Autodesk Inventor part; units mm, degrees
ref_plane "YZ Plane" through (0, 0, 0) normal (1, 0, 0) x (0, 1, 0)
ref_plane "XZ Plane" through (0, 0, 0) normal (0, 1, 0) x (-1, 0, 0)
ref_plane "XY Plane" through (0, 0, 0) normal (0, 0, 1) x (1, 0, 0)
sketch "Skizze1" plane through (0, 0, 0) normal (0, 1, 0) x (-1, 0, 0)
  line L0 (47, -24.5) -> (-47, -24.5)
  line L1 (-47, -24.5) -> (-47, 24.5)
  line L2 (-47, 24.5) -> (47, 24.5)
  line L3 (47, 24.5) -> (47, -24.5)
  point P0 (0, 0)
  point P1 (0, -24.5)
  point P2 (47, 0)
  dimension "d0" = 49
  dimension "d1" = 94
extrude "Extrusion1" add sketch "Skizze1" along normal blind 2
sketch "Skizze2" plane through (0, 2, 0) normal (0, 1, 0) x (1, 0, 0)
  circle A0 centre (-43.5, 21) radius 1.75
  circle A1 centre (-43.5, -21) radius 1.75
  circle A2 centre (43.5, -21) radius 1.75
  circle A3 centre (43.5, 21) radius 1.75
  point P0 (0, 0)
  dimension "d4" = 3.5
  dimension "d5" = 3.5
  dimension "d6" = 3.5
  dimension "d7" = 3.5
  dimension "d8" = 87
  dimension "d9" = 43.5
  dimension "d10" = 42
  dimension "d11" = 21
extrude "Extrusion2" cut sketch "Skizze2" against normal through all
sketch "Skizze4" plane through (0, 2, 0) normal (0, 1, 0) x (1, 0, 0)
  line L0 (-39.5, 24) -> (39.5, 24)
  line L1 (46.5, 17) -> (46.5, -17)
  line L2 (39.5, -24) -> (-39.5, -24)
  line L3 (-46.5, -17) -> (-46.5, 17)
  line L4 (47, -24.5) -> (47, 24.5)
  line L5 (47, 24.5) -> (-47, 24.5)
  line L6 (-47, -24.5) -> (47, -24.5)
  line L7 (-47, 24.5) -> (-47, -24.5)
  circle A0 centre (-43.5, 21) radius 1.75
  arc A1 (-46.5, 17) -> (-39.5, 24) centre (-43.5, 21) ccw
  circle A2 centre (-43.5, -21) radius 1.75
  arc A3 (-39.5, -24) -> (-46.5, -17) centre (-43.5, -21) ccw
  circle A4 centre (43.5, -21) radius 1.75
  arc A5 (46.5, -17) -> (39.5, -24) centre (43.5, -21) ccw
  arc A6 (39.5, 24) -> (46.5, 17) centre (43.5, 21) ccw
  circle A7 centre (43.5, 21) radius 1.75
  point P0 (0, 0)
  dimension "d14" = 0.5
  dimension "d15" = 0.5
  dimension "d16" = 0.5
  dimension "d17" = 0.5
  dimension "d19" = 5
  dimension "d20" = 5
  dimension "d21" = 5
  dimension "d22" = 5
extrude "Extrusion3" add sketch "Skizze4" along normal blind 22 and the other way blind 4 contours L0 A6 L1 A5 L2 A3 L3 A1
equation "\"d14\" = d15"
equation "\"d16\" = d15"
equation "\"d17\" = d15"
equation "\"d19\" = d20"
equation "\"d21\" = d20"
equation "\"d22\" = d20"
properties part number "netzteil_3.3V"
CAD build for the part. Positions are in the model's coordinates, mm. A direction names the side the tool comes from. Round coordinates to 2 decimals unless told otherwise and drop trailing zeros. Loops run counter-clockwise (first coordinate to the right, second up) from the corner with the lowest first, then second, coordinate; pieces in that order, holes last. Notation, with made-up numbers: (19, -36) - (38, -36) arc R14 cw to (38, -20) - close; hole circle Ø9 at (40.5, 54). An arc over 180 degrees is marked (long way). Return JSON: item names as keys, results as strings. Group by question number.
Q1. Band-saw the part on B-B on z = 21. Give the cut face in (x, y), plus the area to 3 significant figures.
Q2. Band-saw the part on D-D on y = 3.75. Give the cut face in (x, z).
Q3. Flat gauge pins, fed straight in: pin 1 Ø3 at (x, z) = (43.5, -21) entering from -Y; pin 2 Ø8 at (x, y) = (-15.5, 15) entering from -Z; pin 3 Ø4 at (y, z) = (12.5, -6) entering from +X; pin 4 Ø12 at (y, z) = (4.5, -1) entering from -X. Where does each tip first touch, or does it go through?
Q4. Band-saw the part on A-A on x = 43.5. Give the cut face in (y, z), plus the area to 3 significant figures.
Q5. Drill centre lines: line 1 along X through (y, z) = (1.4, 21); line 2 along Z through (x, y) = (43.5, 0.95); line 3 along X through (y, z) = (13.75, 16.5). Where is each one in solid material? Low to high. Write a range as [from, to].
Q6. Tool access for faces 1 (the face through (1, 13, 24)), 2 (the face through (40.04, 12.85, -17.39)), 3 (the face through (46.5, -1, 0)), 4 (the face through (-46.5, 13, 0)), 5 (the face through (-46.5, -1, 0)): list every direction of +Z, -Z, +X, -X, +Y, -Y with a clear straight run to the whole face (end or side of a thin tool).
Q7. Band-saw the part on C-C on x = -19. Give the cut face in (y, z), plus the area to 3 significant figures.
Q8. Two-plate mould, pull along Y, no slides. Class faces 6 (the face through (-1, 24, 0)), 7 (the face through (1, -1, 24)), 8 (the face through (-1, -2, 0)): +Y half, -Y half, draft (parallel to the pull), parting line (faces both ways), or undercut.
Solutions:
{
 "1": {"outline": "(-47, 0) - (-45.25, 0) - (-45.25, 2) - (-47, 2) - close; (-41.75, 0) - (-38.5, 0) - (-38.5, -2) - (38.5, -2) - (38.5, 0) - (41.75, 0) - (41.75, 2) - (38.5, 2) - (38.5, 24) - (-38.5, 24) - (-38.5, 2) - (-41.75, 2) - close; (45.25, 0) - (47, 0) - (47, 2) - (45.25, 2) - close", "area": "2,020 mm^2"},
 "2": {"outline": "(-46.5, -17) arc R5 cw to (-39.5, -24) - (39.5, -24) arc R5 cw to (46.5, -17) - (46.5, 17) arc R5 cw to (39.5, 24) - (-39.5, 24) arc R5 cw to (-46.5, 17) - close"},
 "3": {"pin 1": "passes through", "pin 2": "stops at z = -24", "pin 3": "stops at x = 46.5", "pin 4": "stops at x = -47"},
 "4": {"outline": "(-2, -16) - (0, -16) - (0, -19.25) - (2, -19.25) - (2, -16) - (24, -16) - (24, 16) - (2, 16) - (2, 19.25) - (0, 19.25) - (0, 16) - (-2, 16) - close; (0, -24.5) - (2, -24.5) - (2, -22.75) - (0, -22.75) - close; (0, 22.75) - (2, 22.75) - (2, 24.5) - (0, 24.5) - close", "area": "852 mm^2"},
 "5": {"line 1": "x = [-47, -45.25], [-41.75, 41.75], [45.25, 47]", "line 2": "z = [-24.5, -22.75], [-19.25, 19.25], [22.75, 24.5]", "line 3": "x = [-46.5, -45.68], [-41.32, 41.32], [45.68, 46.5]"},
 "6": {"face 1": "+Z, +X, -X, +Y", "face 2": "+Y", "face 3": "+Z, -Z, +X, -Y", "face 4": "+Z, -Z, -X, +Y", "face 5": "+Z, -Z, -X, -Y"},
 "7": {"outline": "(-2, -24) - (0, -24) - (0, -24.5) - (2, -24.5) - (2, -24) - (24, -24) - (24, 24) - (2, 24) - (2, 24.5) - (0, 24.5) - (0, 24) - (-2, 24) - close", "area": "1,250 mm^2"},
 "8": {"face 6": "+Y half", "face 7": "draft", "face 8": "-Y half"}
}
